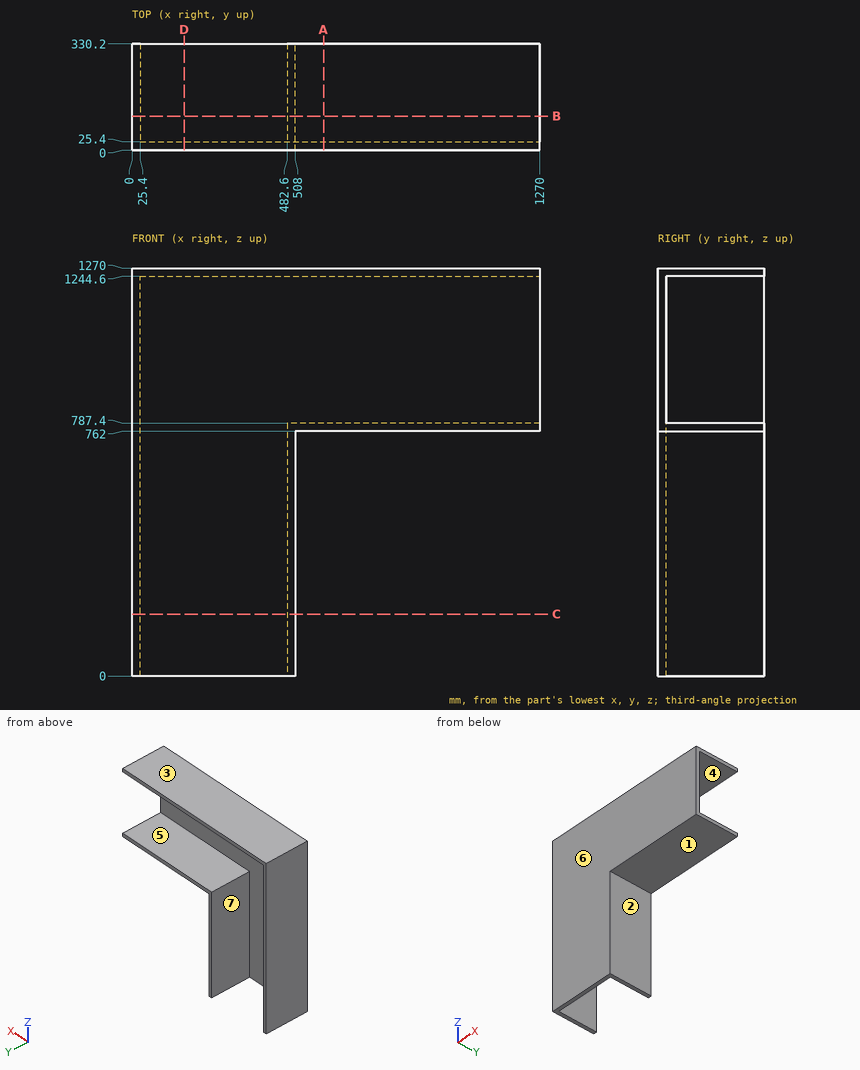
For this review, use the dimensioned drawing (mm, ordinates from the lowest corner) and the shaded views. A direction names the side the tool comes from. Round coordinates to 2 decimals unless told otherwise and drop trailing zeros. Order: outer loops, then holes, each group sorted by start corner. A loop starts at its lowest first (then second) coordinate and runs counter-clockwise, first axis right, second up. Notation, with made-up numbers: M -21.5,-1 L 11.5,-1 A32 ccw 11.5,26 Z; hole C -1,39 d5. An arc over 180 degrees is marked long. Use a Markdown table: item, result.
1) Consider section C-C (z = 193). Write out the cut boundary in (x, y), then the cut area to 3 significant figures.
Report:
| item | result |
|---|---|
| outline | M 0,0 L 508,0 L 508,330.2 L 482.6,330.2 L 482.6,25.4 L 25.4,25.4 L 25.4,330.2 L 0,330.2 Z |
| area | 28,400 mm^2 |
2) Tool access review of the marked faces 5, 6 and 7: name each direction out of +Z, -Z, +X, -X, +Y, -Y from which nothing blocks a thin tool from reaching the whole face with its end or side.
Report:
| item | result |
|---|---|
| face 5 | +X, +Y |
| face 6 | +Z, -Z, +X, -X, -Y |
| face 7 | -Z, +Y |
3) Consider section A-A (x = 596.5). Write out the cut boundary in (y, z).
Report:
| item | result |
|---|---|
| outline | M 0,762 L 330.2,762 L 330.2,787.4 L 25.4,787.4 L 25.4,1244.6 L 330.2,1244.6 L 330.2,1270 L 0,1270 Z |
4) Consider section D-D (x = 162). Write out the cut boundary in (y, z), then the cut area to 3 significant figures.
Report:
| item | result |
|---|---|
| outline | M 0,0 L 25.4,0 L 25.4,1244.6 L 330.2,1244.6 L 330.2,1270 L 0,1270 Z |
| area | 40,000 mm^2 |
5) Draft analysis for pull direction Z (two halves, no side actions). For the marked faces 1, 2, 3 and 4, state which applies: released by +Z, released by -Z, zero draft, split by the parting line, or undercut.
Report:
| item | result |
|---|---|
| face 1 | released by -Z |
| face 2 | zero draft |
| face 3 | released by +Z |
| face 4 | undercut |
6) Consider section B-B (y = 105.5). Write out the cut boundary in (x, z).
Report:
| item | result |
|---|---|
| outline | M 0,0 L 25.4,0 L 25.4,1244.6 L 1270,1244.6 L 1270,1270 L 0,1270 Z; M 482.6,0 L 508,0 L 508,762 L 1270,762 L 1270,787.4 L 482.6,787.4 Z |
7) Insertion check: pin 1 (2 mm diameter, centred on y = 87, z = 1046.5, fed in from -X); pin 2 (1 mm diameter, centred on y = 264, z = 323, fed in from +X); pin 3 (12 mm diameter, centred on x = 345.5, z = 1123, fed in from +Y). Each pin has a flat end and moves straight along its axis. Give the tip position at first contact, or say it passes through.
Report:
| item | result |
|---|---|
| pin 1 | x = 0 |
| pin 2 | x = 508 |
| pin 3 | y = 25.4 |
8) Wall thickness on line 1 along Z through (x, y) = (708, 61); line 2 along Z through (x, y) = (505, 180.5); line 3 along X through (y, z) = (231.5, 302): over which ranges is each line inside the solid? List them lowest first. Write a range as [from, to].
Report:
| item | result |
|---|---|
| line 1 | [762, 787.4], [1244.6, 1270] |
| line 2 | [0, 787.4], [1244.6, 1270] |
| line 3 | [0, 25.4], [482.6, 508] |
